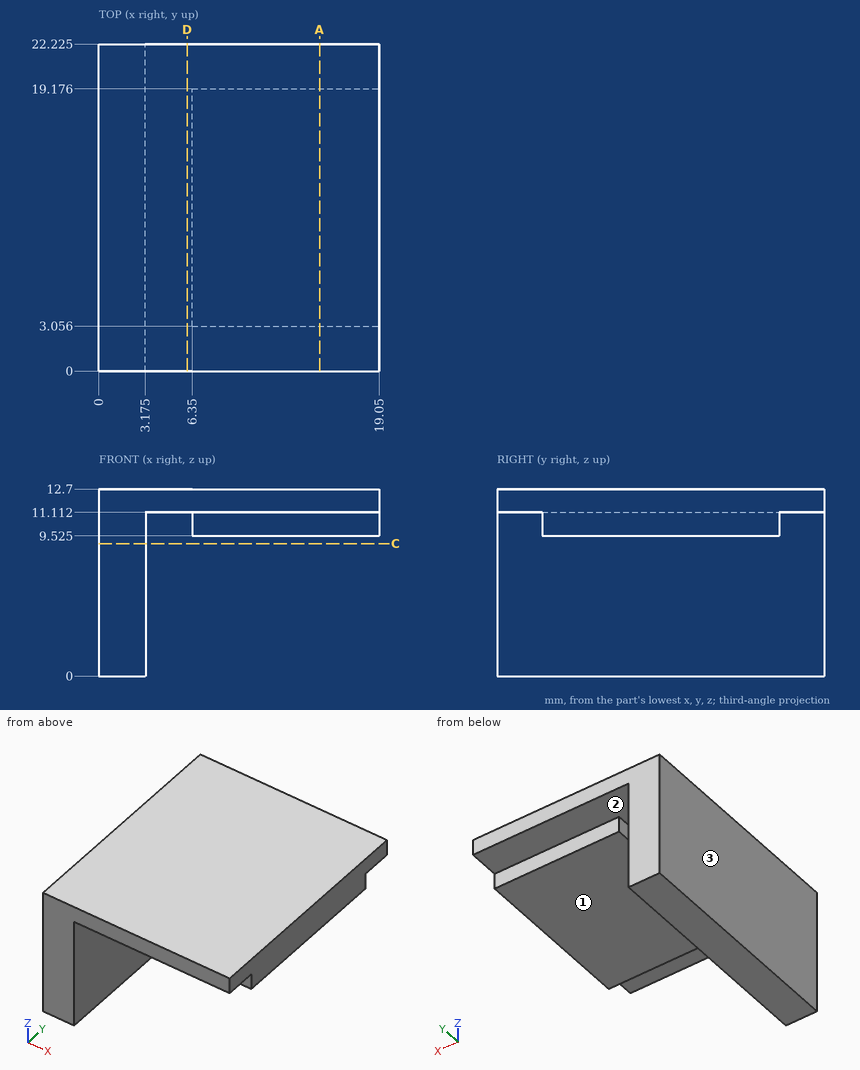
Source: three-view drawing plus pictorial views. Frame: mm from the lowest corner of the part. Give positions to 0.01 mm unless a question says otherwise; leave off trailing zeros. Order: outer loops, then holes, each group sorted by start corner. A loop starts at its lowest first (then second) coordinate and runs counter-clockwise, first axis right, second up. Notation, with made-up numbers: M -22.5,75 L 27.5,75 A21 cw 27.5,101 Z; hole C -6.75,72.25 d4. An arc over 180 degrees is marked long. One line per question, with ' | ' between items. Start each with the question number.
1. Pull-direction query (X, two-part tool) for the marked faces 1, 2 and 3; classes: released by +X, released by -X, zero draft, split by the parting line, or undercut.
2. Section query C-C (z = 9). Return the cut outline in (x, y) (1 decimal).
3. Section query D-D (x = 6). Return the cut outline in (y, z) (1 decimal).
4. Material intervals for probe 1 along Z at (x, y) = (17, 18.25) (1 decimal); probe 2 along X at (y, z) = (13.25, 1.5) (1 decimal); probe 3 along Y at (x, z) = (9.5, 9.75) (1 decimal), sorted ascending. Write a range as [from, to].
5. First-contact query: pin 1 Ø10 at (x, y) = (15.5, 14.5) entering from -Z (1 decimal); pin 2 Ø0.5 at (x, z) = (9.5, 10.5) entering from -Y (1 decimal); pin 3 Ø3.5 at (y, z) = (12, 6) entering from +X (1 decimal). Flat tips, straight axial feed; report the tip coordinate or a pass-through.
6. Section query A-A (x = 15). Return the cut outline in (y, z) (1 decimal).
Here are the results:
1) face 1: zero draft | face 2: undercut | face 3: released by -X
2) outline: M 0,0 L 3.2,0 L 3.2,22.2 L 0,22.2 Z
3) outline: M 0,11.1 L 22.2,11.1 L 22.2,12.7 L 0,12.7 Z
4) probe 1: [9.5, 12.7] | probe 2: [0, 3.2] | probe 3: [3.1, 19.2]
5) pin 1: z = 9.5 | pin 2: y = 3.1 | pin 3: x = 3.2
6) outline: M 0,11.1 L 3.1,11.1 L 3.1,9.5 L 19.2,9.5 L 19.2,11.1 L 22.2,11.1 L 22.2,12.7 L 0,12.7 Z
